from build123d import *

# Parameters (mm, degrees)
F1_DEPTH = 10
F2_T     = -1
F3_R     = 12.840511
F4_DEPTH = 25


with BuildPart() as f1:
    # F0 (on Top) → F1 (new body)
    with BuildSketch(Plane.XY):
        with BuildLine():
            Line((-4.188098, 34.173166), (-64.188098, 34.173166))
            ThreePointArc((-64.188098, 34.173166), (-74.7947, 29.779768), (-79.188098, 19.173166))
            Line((-79.188098, 19.173166), (-79.188098, -40.826834))
            ThreePointArc((-79.188098, -40.826834), (-74.7947, -51.433435), (-64.188098, -55.826834))
            ThreePointArc((-64.188098, -55.826834), (-53.581496, -51.433435), (-49.188098, -40.826834))
            Line((-49.188098, -40.826834), (-49.188098, -10.826834))
            ThreePointArc((-49.188098, -10.826834), (-44.7947, -0.220232), (-34.188098, 4.173166))
            ThreePointArc((-34.188098, 4.173166), (-23.581496, -0.220232), (-19.188098, -10.826834))
            Line((-19.188098, -10.826834), (-19.188098, -40.826834))
            ThreePointArc((-19.188098, -40.826834), (-14.7947, -51.433435), (-4.188098, -55.826834))
            ThreePointArc((-4.188098, -55.826834), (6.418504, -51.433435), (10.811902, -40.826834))
            Line((10.811902, -40.826834), (10.811902, 19.173166))
            ThreePointArc((10.811902, 19.173166), (6.418504, 29.779768), (-4.188098, 34.173166))
        make_face()
    extrude(amount=F1_DEPTH)

    # F2
    f2_openings = [f1.faces().sort_by_distance(p)[0] for p in [
        (-4.188098, -54.554042, 10),
    ]]
    offset(amount=F2_T, openings=f2_openings)

    # F3 (on face) → F4 (cut)
    with BuildSketch(Plane.XY.offset(1)):
        with Locations((-64.188098, 19.173166)):
            Circle(F3_R)
    extrude(amount=-F4_DEPTH, mode=Mode.SUBTRACT)


solid = f1.part
Check sheet for the modelled part. Datum: model origin and axes. Units: mm. A direction names the side the tool comes from. Coordinates: 2 decimals unless noted, no trailing zeros. Write each loop counter-clockwise with the first axis right and the second up, starting at its lowest first coordinate (ties: lowest second). Pieces come first, ordered by that corner, then holes.
Item 1: Access from +Z, -Z, +X, -X, +Y, -Y to the whole of each face (thin tool, end or side, straight path). Record for faces 1 (the face through (-73.98, 29.18, 5.44)), 2 (the face through (-45, 0, 0)), 3 (the face through (-49.188, -26, 5)).
Numbers:
face 1: +Z
face 2: -Z, +X, -X, +Y, -Y
face 3: +Z, -Z, -Y
Item 2: Cross-section at B-B on x = -69. Record the boundary of the cut face in (y, z), then the cut area to 3 significant figures.
Numbers:
outline: (-55.03, 0) - (7.27, 0) - (7.27, 1) - (-53.97, 1) - (-53.97, 10) - (-55.03, 10) - close; (31.08, 0) - (33.38, 0) - (33.38, 10) - (32.32, 10) - (32.32, 1) - (31.08, 1) - close
area: 83.7 mm2
Item 3: Cross-section at C-C on z = 5.75. Record the boundary of the cut face in (x, y).
Numbers:
outline: (-79.19, -40.83) arc R15 ccw to (-64.19, -55.83) arc R15 ccw to (-49.19, -40.83) - (-49.19, -10.83) arc R15 cw to (-34.19, 4.17) arc R15 cw to (-19.19, -10.83) - (-19.19, -40.83) arc R15 ccw to (-4.19, -55.83) arc R15 ccw to (10.81, -40.83) - (10.81, 19.17) arc R15 ccw to (-4.19, 34.17) - (-64.19, 34.17) arc R15 ccw to (-79.19, 19.17) - close; hole (-78.19, -40.83) arc R14 ccw to (-64.19, -54.83) arc R14 ccw to (-50.19, -40.83) - (-50.19, -10.83) arc R16 cw to (-34.19, 5.17) arc R16 cw to (-18.19, -10.83) - (-18.19, -40.83) arc R14 ccw to (-4.19, -54.83) arc R14 ccw to (9.81, -40.83) - (9.81, 19.17) arc R14 ccw to (-4.19, 33.17) - (-64.19, 33.17) arc R14 ccw to (-78.19, 19.17) - close
Item 4: Cross-section at A-A on y = -36. Record the boundary of the cut face in (x, z), then the cut area to 3 significant figures.
Numbers:
outline: (-79.19, 0) - (-49.19, 0) - (-49.19, 10) - (-50.19, 10) - (-50.19, 1) - (-78.19, 1) - (-78.19, 10) - (-79.19, 10) - close; (-19.19, 0) - (10.81, 0) - (10.81, 10) - (9.81, 10) - (9.81, 1) - (-18.19, 1) - (-18.19, 10) - (-19.19, 10) - close
area: 96.0 mm2
Item 5: Scan lines: probe 1 along X at (y, z) = (-37, 2.75); probe 2 along X at (y, z) = (-9, 1.75); probe 3 along X at (y, z) = (8.5, 5.75). Record each from-to range of solid material in increasing order.
Numbers:
probe 1: x = -79.19 to -78.19, -50.19 to -49.19, -19.19 to -18.19, 9.81 to 10.81
probe 2: x = -79.19 to -78.19, -50.08 to -49.08, -19.3 to -18.29, 9.81 to 10.81
probe 3: x = -79.19 to -78.19, 9.81 to 10.81
Item 6: Depth check by flat-ended pin: pin 1 Ø2 at (y, z) = (22, 4.5) entering from +X; pin 2 Ø5 at (x, y) = (-22.5, 11) entering from -Z. Enter the tip coordinate at first touch or a pass-through.
Numbers:
pin 1: stops at x = 10.7
pin 2: stops at z = 0
Item 7: Cross-section at D-D on x = -22. Record the boundary of the cut face in (y, z).
Numbers:
outline: (-2.08, 0) - (34.17, 0) - (34.17, 10) - (33.17, 10) - (33.17, 1) - (-0.46, 1) - (-0.46, 10) - (-2.08, 10) - close
Item 8: Mould release check, pull along Y, two halves, no side actions. Record for faces 4 (the face through (-18.188, -26, 5)), 5 (the face through (-48, -4, 10)), 6 (the face through (6.5, 29.7, 4.9)): released by +Y, released by -Y, zero draft, split by the parting line, or undercut.
Numbers:
face 4: undercut
face 5: zero draft
face 6: released by +Y
